```python
from build123d import *

# Parameters (mm, degrees)
EXTRUDE_1_DEPTH      = 26
CUT_EXTRUDE_START    = -10
CUT_EXTRUDE_1_DEPTH  = 10
SKETCH_3_W           = 3
SKETCH_3_H           = 8.5
EXTRUDE_2_DEPTH      = 3
CUT_EXTRUDE_2_REACH  = 37.412
SKETCH_5_W           = 3
SKETCH_5_H           = 8.5
EXTRUDE_3_DEPTH      = 3
CUT_EXTRUDE_3_REACH  = 37.412
SKETCH_7_W           = 11
SKETCH_7_H           = 20
CUT_EXTRUDE_4_DEPTH  = 2
FILLET_3_R           = 1
FILLET_4_R           = 1
SKETCH_10_W          = 15
SKETCH_10_H          = 7
CUT_EXTRUDE_5_DEPTH  = 2
CUT_EXTRUDE_START_2  = -4
CUT_EXTRUDE_6_DEPTH  = 4
FILLET_5_R           = 0.5
FILLET_6_R           = 0.5
FILLET_7_R           = 1
FILLET_9_R           = 0.7
FILLET_10_R          = 0.7
SKETCH_12_W          = 3
SKETCH_12_H          = 4
CUT_EXTRUDE_7_DEPTH  = 4
FILLET_11_R          = 1.5
FILLET_12_R          = 0.5
SKETCH_13_R          = 2.75
CUT_EXTRUDE_16_DEPTH = 10
SKETCH_14_W          = 17
SKETCH_14_H          = 3
CUT_EXTRUDE_20_DEPTH = 15
FILLET_13_R          = 0.7
SKETCH_15_W          = 1.5
SKETCH_15_H          = 2
CUT_EXTRUDE_22_DEPTH = 15


with BuildPart() as part:
    # ｽｹｯﾁ1 → ﾎﾞｽ - 押し出し1 (new body)
    with BuildSketch(Plane.XY):
        with BuildLine():
            Line((8.5, -8.5), (-8.5, -8.5))
            ThreePointArc((-8.5, -8.5), (-17, 0), (-8.5, 8.5))
            Line((-8.5, 8.5), (8.5, 8.5))
            ThreePointArc((8.5, 8.5), (17, 0), (8.5, -8.5))
        make_face()
    extrude(amount=EXTRUDE_1_DEPTH)

    # ｽｹｯﾁ2 → ｶｯﾄ - 押し出し1 (cut)
    with BuildSketch(Plane.XY.offset(26).offset(CUT_EXTRUDE_START)):
        with BuildLine():
            Line((-8.5, 8.5), (-8.5, -8.5))
            ThreePointArc((-8.5, -8.5), (-17, 0), (-8.5, 8.5))
        make_face()
        with BuildLine():
            Line((8.5, 8.5), (8.5, -8.5))
            ThreePointArc((8.5, -8.5), (17, 0), (8.5, 8.5))
        make_face()
    extrude(amount=CUT_EXTRUDE_1_DEPTH, mode=Mode.SUBTRACT)

    # ｽｹｯﾁ3 → ﾎﾞｽ - 押し出し2 (add)
    with BuildSketch(Plane(origin=(8.5, 0, 0), x_dir=(0, 0, -1), z_dir=(1, 0, 0))):
        with Locations((-24.5, 4.25)):
            Rectangle(SKETCH_3_W, SKETCH_3_H)
    extrude(amount=EXTRUDE_2_DEPTH)

    # ｽｹｯﾁ4 → ｶｯﾄ - 押し出し2 (cut, up to next)
    with BuildSketch(Plane(origin=(0, 8.5, 0), x_dir=(1, 0, 0), z_dir=(0, 1, 0)), mode=Mode.PRIVATE) as cut_extrude_2_sk1:
        Polygon((11.5, -23), (11.5, -26), (8.5, -26), align=None)
    cut_extrude_2_tool1 = extrude(cut_extrude_2_sk1.sketch, amount=-CUT_EXTRUDE_2_REACH, mode=Mode.PRIVATE) & part.part
    add(cut_extrude_2_tool1.solids().sort_by_distance((10.5, 8.5, 25))[0], mode=Mode.SUBTRACT)

    # ｽｹｯﾁ5 → ﾎﾞｽ - 押し出し3 (add)
    with BuildSketch(Plane.ZY.offset(8.5)):
        with Locations((24.5, 4.25)):
            Rectangle(SKETCH_5_W, SKETCH_5_H)
    extrude(amount=EXTRUDE_3_DEPTH)

    # ｽｹｯﾁ6 → ｶｯﾄ - 押し出し3 (cut, up to next)
    with BuildSketch(Plane(origin=(0, 8.5, 0), x_dir=(1, 0, 0), z_dir=(0, 1, 0)), mode=Mode.PRIVATE) as cut_extrude_3_sk1:
        Polygon((-11.5, -26), (-11.5, -23), (-8.5, -26), align=None)
    cut_extrude_3_tool1 = extrude(cut_extrude_3_sk1.sketch, amount=-CUT_EXTRUDE_3_REACH, mode=Mode.PRIVATE) & part.part
    add(cut_extrude_3_tool1.solids().sort_by_distance((-10.5, 8.5, 25))[0], mode=Mode.SUBTRACT)

    # ｽｹｯﾁ7 → ｶｯﾄ - 押し出し4 (cut)
    with BuildSketch(Plane.XZ.offset(8.5)):
        with Locations((0, 13)):
            Rectangle(SKETCH_7_W, SKETCH_7_H)
    extrude(amount=-CUT_EXTRUDE_4_DEPTH, mode=Mode.SUBTRACT)

    # ﾌｨﾚｯﾄ3
    fillet_3_edges = [part.edges().sort_by_distance(p)[0] for p in [
        (5.5, -7.5, 3),
    ]]
    fillet(fillet_3_edges, radius=FILLET_3_R)

    # ﾌｨﾚｯﾄ4
    fillet_4_edges = [part.edges().sort_by_distance(p)[0] for p in [
        (-5.5, -7.5, 3),
    ]]
    fillet(fillet_4_edges, radius=FILLET_4_R)

    # ｽｹｯﾁ10 → ｶｯﾄ - 押し出し5 (cut)
    with BuildSketch(Plane.XZ.offset(8.5)):
        with Locations((0, 19.5)):
            Rectangle(SKETCH_10_W, SKETCH_10_H)
    extrude(amount=-CUT_EXTRUDE_5_DEPTH, mode=Mode.SUBTRACT)

    # ｽｹｯﾁ11 → ｶｯﾄ - 押し出し6 (cut)
    with BuildSketch(Plane.XZ.offset(8.5).offset(CUT_EXTRUDE_START_2)):
        with BuildLine():
            Line((6.5, 21), (3.5, 21))
            Line((3.5, 21), (3.5, 5))
            Line((3.5, 5), (0, 5))
            Line((0, 5), (0, 3.001563835))
            Line((0, 3.001563835), (4.5, 3))
            ThreePointArc((4.5, 3), (5.207106781, 3.292893219), (5.5, 4))
            Line((5.5, 4), (5.5, 16))
            Line((5.5, 16), (6.5, 16))
            Line((6.5, 16), (6.5, 21))
        make_face()
    cut_extrude_6 = extrude(amount=CUT_EXTRUDE_6_DEPTH, mode=Mode.SUBTRACT)

    # ﾐﾗｰ1: ｶｯﾄ - 押し出し6 across plane
    add(cut_extrude_6.mirror(Plane(origin=(0, 0, 0), x_dir=(0, 0, 1), z_dir=(1, 0, 0))), mode=Mode.SUBTRACT)

    # ﾌｨﾚｯﾄ5
    fillet_5_edges = [part.edges().sort_by_distance(p)[0] for p in [
        (3.5, -5.5, 5),
    ]]
    fillet(fillet_5_edges, radius=FILLET_5_R)

    # ﾌｨﾚｯﾄ6
    fillet_6_edges = [part.edges().sort_by_distance(p)[0] for p in [
        (-3.5, -5.5, 5),
    ]]
    fillet(fillet_6_edges, radius=FILLET_6_R)

    # ﾌｨﾚｯﾄ7
    fillet_7_edges = [part.edges().sort_by_distance(p)[0] for p in [
        (3.5, -5.5, 21),
        (6.5, -5.5, 21),
        (-6.5, -5.5, 21),
        (-3.5, -5.5, 21),
    ]]
    fillet(fillet_7_edges, radius=FILLET_7_R)

    # ﾌｨﾚｯﾄ9
    fillet_9_edges = [part.edges().sort_by_distance(p)[0] for p in [
        (-11.5, 4.25, 23),
    ]]
    fillet(fillet_9_edges, radius=FILLET_9_R)

    # ﾌｨﾚｯﾄ10
    fillet_10_edges = [part.edges().sort_by_distance(p)[0] for p in [
        (11.5, 4.25, 23),
    ]]
    fillet(fillet_10_edges, radius=FILLET_10_R)

    # ｽｹｯﾁ12 → ｶｯﾄ - 押し出し7 (cut)
    with BuildSketch(Plane.XZ.offset(8.5)):
        with Locations((0, 9)):
            Rectangle(SKETCH_12_W, SKETCH_12_H)
    extrude(amount=-CUT_EXTRUDE_7_DEPTH, mode=Mode.SUBTRACT)

    # ﾌｨﾚｯﾄ11
    fillet_11_edges = [part.edges().sort_by_distance(p)[0] for p in [
        (0, -6.5, 23),
    ]]
    fillet(fillet_11_edges, radius=FILLET_11_R)

    # ﾌｨﾚｯﾄ12
    fillet_12_edges = [part.edges().sort_by_distance(p)[0] for p in [
        (0, -8.5, 23),
    ]]
    fillet(fillet_12_edges, radius=FILLET_12_R - 0.0001)  # a hair under: the kernel refuses the full size

    # ｽｹｯﾁ13 → ｶｯﾄ - 押し出し16 (cut)
    with BuildSketch(Plane.XY.offset(26)):
        Circle(SKETCH_13_R)
        with Locations((-5.7, 0)):
            Circle(SKETCH_13_R)
        with Locations(Location((5.7, 0, 0), (0, 0, 180))):
            Circle(SKETCH_13_R)
    extrude(amount=-CUT_EXTRUDE_16_DEPTH, mode=Mode.SUBTRACT)

    # ｽｹｯﾁ14 → ｶｯﾄ - 押し出し20 (cut)
    with BuildSketch(Plane(origin=(0, 0, 0), x_dir=(-1, 0, 0), z_dir=(0, 0, -1))):
        with BuildLine():
            Line((8.5, -6), (-8.5, -6))
            ThreePointArc((-8.5, -6), (-14.5, 0), (-8.5, 6))
            Line((-8.5, 6), (8.5, 6))
            ThreePointArc((8.5, 6), (14.5, 0), (8.5, -6))
        make_face()
        Rectangle(SKETCH_14_W, SKETCH_14_H, mode=Mode.SUBTRACT)
    extrude(amount=-CUT_EXTRUDE_20_DEPTH, mode=Mode.SUBTRACT)

    # ﾌｨﾚｯﾄ13
    fillet_13_edges = [part.edges().sort_by_distance(p)[0] for p in [
        (8.5, 1.5, 7.5),
        (-8.5, 1.5, 7.5),
        (-8.5, -1.5, 7.5),
        (8.5, -1.5, 7.5),
    ]]
    fillet(fillet_13_edges, radius=FILLET_13_R)

    # ｽｹｯﾁ15 → ｶｯﾄ - 押し出し22 (cut)
    with BuildSketch(Plane(origin=(0, 0, 0), x_dir=(-1, 0, 0), z_dir=(0, 0, -1))):
        with Locations((-6.75, 0)):
            Rectangle(SKETCH_15_W, SKETCH_15_H)
        with Locations((6.75, 0)):
            Rectangle(SKETCH_15_W, SKETCH_15_H)
        Rectangle(SKETCH_15_W, SKETCH_15_H)
    extrude(amount=-CUT_EXTRUDE_22_DEPTH, mode=Mode.SUBTRACT)


solid = part.part
```
Input: part model. Units: mm. Frame: model coordinates. A direction names the side the tool comes from. Give positions to 0.01 mm unless a question says otherwise; leave off trailing zeros. Order: outer loops, then holes, each group sorted by start corner. A loop starts at its lowest first (then second) coordinate and runs counter-clockwise, first axis right, second up. Notation, with made-up numbers: (-36.75, -34) - (17.25, -34) arc R14 ccw to (17.25, -20) - close; hole circle Ø1 at (-33.5, -34.75). An arc over 180 degrees is marked (long way). Use a Markdown table: item, result.
(1) Section query C-C (y = -2). Output: boundary loops of the cut face in (x, z).
Computed values:
| item | result |
|---|---|
| outline | (-16.76, 0) - (-14.16, 0) - (-14.16, 15) - (14.16, 15) - (14.16, 0) - (16.76, 0) - (16.76, 16) - (8.5, 16) - (8.5, 26) - (7.59, 26) - (7.59, 16) - (3.81, 16) - (3.81, 26) - (1.89, 26) - (1.89, 16) - (-1.89, 16) - (-1.89, 26) - (-3.81, 26) - (-3.81, 16) - (-7.59, 16) - (-7.59, 26) - (-8.5, 26) - (-8.5, 16) - (-16.76, 16) - close |
(2) Draft query along Y for faces 1 (the cylindrical face through (-3.16, -1.05, 21.07)), 2 (the flat face through (-5, -5, 21)), 3 (the flat face through (9, 0, 24)). Return one class per face: released by +Y, released by -Y, zero draft, split by the parting line, or undercut.
Computed values:
| item | result |
|---|---|
| face 1 | undercut |
| face 2 | zero draft |
| face 3 | released by -Y |
(3) Line query: line 1 (Y direction, x = 0, z = 2.25); line 2 (X direction, y = 0, z = 6.75); line 3 (Y direction, x = -5.7, z = 19). Output: solid intervals per line, ascending. Write a range as from..to.
Computed values:
| item | result |
|---|---|
| line 1 | y = -8.5..-6, -1.5..-1, 1..1.5, 6..8.5 |
| line 2 | x = -17..-14.5, -8.5..-7.5, -6..-0.75, 0.75..6, 7.5..8.5, 14.5..17 |
| line 3 | y = -4.5..-2.75, 2.75..8.5 |
(4) Section query D-D (x = -12). Output: boundary loops of the cut face in (y, z), then the cut area to 3 significant figures.
Computed values:
| item | result |
|---|---|
| outline | (-7.75, 0) - (-4.87, 0) - (-4.87, 15) - (4.87, 15) - (4.87, 0) - (7.75, 0) - (7.75, 16) - (-7.75, 16) - close |
| area | 102 mm2 |
(5) Section query A-A (z = 18.25). Output: boundary loops of the cut face in (x, y).
Computed values:
| item | result |
|---|---|
| outline | (-8.5, -8.5) - (-7.5, -8.5) - (-7.5, -6.5) - (-6.5, -6.5) - (-6.5, -4.5) - (-3.5, -4.5) - (-3.5, -6.5) - (3.5, -6.5) - (3.5, -4.5) - (6.5, -4.5) - (6.5, -6.5) - (7.5, -6.5) - (7.5, -8.5) - (8.5, -8.5) - (8.5, 8.5) - (-8.5, 8.5) - close; hole circle Ø5.5 at (-5.7, 0); hole circle Ø5.5 at (0, 0); hole circle Ø5.5 at (5.7, 0) |
(6) Section query B-B (z = 13.5). State how many separate pieces and enclosed holes the cut face has, then the cut area to 3 significant figures.
Computed values:
| item | result |
|---|---|
| separate pieces | 3 |
| enclosed holes | 3 |
| area | 216 mm2 |
(7) Pin query (flat end, axial travel): pin 1 (1.5 mm diameter, centred on y = -5.5, z = 13.5, fed in from +X); pin 2 (0.9 mm diameter, centred on x = 4.5, z = 17.5, fed in from -Y); pin 3 (2 mm diameter, centred on x = -3.5, z = 20.5, fed in from -Y). Return the tip coordinate at first contact, or that it passes through.
Computed values:
| item | result |
|---|---|
| pin 1 | stops at x = 15.55 |
| pin 2 | stops at y = -4.5 |
| pin 3 | stops at y = -6.5 |
(8) Access query for faces 4 (the flat face through (6, 0, 16)), 5 (the cylindrical face through (5.199, -7.232, 3.285)), 6 (the cylindrical face through (14.5, -0.1, 7.4)). Directions: +Z, -Z, +X, -X, +Y, -Y. A direction counts if a zero-diameter tool reaches every point of the face in a straight line with its end or side. Return the directions, or none.
Computed values:
| item | result |
|---|---|
| face 4 | +Z |
| face 5 | -Y |
| face 6 | -Z |
